Part model, mm, in its own coordinate system. A direction names the side the tool comes from. Round coordinates to 2 decimals unless told otherwise and drop trailing zeros. Write each loop counter-clockwise with the first axis right and the second up, starting at its lowest first coordinate (ties: lowest second). Pieces come first, ordered by that corner, then holes. Notation, with made-up numbers: (21.25, -6) -> (50.25, -6) arc R10 ccw to (50.25, -1) -> close; hole circle Ø5 at (18, 79). An arc over 180 degrees is marked (long way). Use CSV: the item, a comma, the result in double quotes. Start each with the question number.
(1) Saw through at A-A (z = 21.5). Give the cut face in (x, y), plus the area to 3 significant figures.
(2) Saw through at D-D (x = 0). Give the cut face in (y, z), plus the area to 3 significant figures.
(3) Two-plate mould, pull along X, no slides. Class faces 1 (the cylindrical face through (-21.664, -4.715, 12.325)), 2 (the flat face through (-25, 3, 12)), 3 (the flat face through (-0.3, -0.4, 25)): released by +X, released by -X, zero draft, split by the parting line, or undercut.
(4) Saw through at B-B (x = -20). Give the cut face in (y, z).
(5) Probe line 1 (Y direction, x = -20, z = 6.25); line 2 (X direction, y = -1.75, z = 2); line 3 (X direction, y = 3, z = 6.5). List the from-to ranges inside material, lowest first. Write a range as [from, to].
(6) Saw through at C-C (y = -1.75). Give the cut face in (x, z), plus the area to 3 significant figures.
(7) Which spindle directions (+Z, -Z, +X, -X, +Y, -Y) get a long thin tool onto all of the face, cutting with end or side? Do faces 4 (the cylindrical face through (0, -5, 15)), 5 (the cylindrical face through (0, -5, 17)), 6 (the flat face through (15, 3, 21)), 7 (the cylindrical face through (0, -7, 19)). Say none if no direction does.
(8) Drop flat-ended pins along their axis: pin 1 (2 mm diameter, centred on x = 3, y = 4.5, fed in from +Z); pin 2 (3.5 mm diameter, centred on x = -4, z = 20, fed in from +Y). Give the stop position or say it passes through.
```python
from build123d import *

# Parameters (mm, degrees)
F0_R          = 3.25
F1_DEPTH      = 25
F3_DEPTH      = 8
F4_START      = 6
F4_DEPTH      = 2
F6_DEPTH      = 25
F7_R          = 1.75
F8_DEPTH      = 25
F8_DEPTH_BACK = 25
F9_R          = 1


with BuildPart() as f1:
    # F0 (on Top) → F1 (new body)
    with BuildSketch(Plane.XY):
        with BuildLine():
            Line((-25, 6.5), (-25, 0))
            ThreePointArc((-25, 0), (-21.5811388301, -4.7434164903), (-16, -3))
            Line((-16, -3), (0, -3))
            Line((0, -3), (16, -3))
            ThreePointArc((16, -3), (21.5811388301, -4.7434164903), (25, 0))
            Line((25, 0), (25, 6.5))
            Line((25, 6.5), (-25, 6.5))
        make_face()
        with Locations((-20, 0)):
            Circle(F0_R, mode=Mode.SUBTRACT)
        with Locations((20, 0)):
            Circle(F0_R, mode=Mode.SUBTRACT)
    extrude(amount=F1_DEPTH)

    # F2 (on Front) → F3 (join)
    with BuildSketch(Plane.XZ):
        with BuildLine():
            ThreePointArc((-8, 10), (0, 15), (8, 10))
            Line((8, 10), (9.797752809, 10.8764044944))
            ThreePointArc((9.797752809, 10.8764044944), (0, 17), (-9.797752809, 10.8764044944))
            Line((-9.797752809, 10.8764044944), (-8, 10))
        make_face()
    extrude(amount=F3_DEPTH)

    # F2 (on Front) → F4 (join)
    with BuildSketch(Plane.XZ.offset(F4_START)):
        with BuildLine():
            ThreePointArc((-9.797752809, 10.8764044944), (0, 17), (9.797752809, 10.8764044944))
            Line((9.797752809, 10.8764044944), (11.595505618, 11.7528089888))
            ThreePointArc((11.595505618, 11.7528089888), (0, 19), (-11.595505618, 11.7528089888))
            Line((-11.595505618, 11.7528089888), (-9.797752809, 10.8764044944))
        make_face()
    extrude(amount=F4_DEPTH)

    # F5 (on Front) → F6 (cut)
    with BuildSketch(Plane.XZ):
        Polygon((-15, 18), (0, 18), (15, 18), (15, 26), (-15, 26), align=None)
    extrude(amount=-F6_DEPTH, mode=Mode.SUBTRACT)

    # F7 (on Front) → F8 (cut, two sides)
    with BuildSketch(Plane.XZ) as f8_sk:
        with Locations((-12, 21.5)):
            Circle(F7_R)
        with Locations((12, 21.5)):
            Circle(F7_R)
    extrude(amount=-F8_DEPTH, mode=Mode.SUBTRACT)
    extrude(f8_sk.sketch, amount=F8_DEPTH_BACK, mode=Mode.SUBTRACT)

    # F9
    f9_edges = [f1.edges().sort_by_distance(p)[0] for p in [
        (0, -3, 15),
        (-8.898876, -3, 10.438202),
        (8.898876, -3, 10.438202),
        (0, -3, 17),
        (0, -8, 15),
    ]]
    fillet(f9_edges, radius=F9_R)


solid = f1.part
```
Answers:
1,outline,"(-25, 0) arc R5 ccw to (-16, -3) -> (-13.75, -3) -> (-13.75, 0) -> (-15, 0) -> (-15, 6.5) -> (-25, 6.5) -> close; (-10.25, -3) -> (10.25, -3) -> (10.25, 0) -> (-10.25, 0) -> close; (13.75, -3) -> (16, -3) arc R5 ccw to (25, 0) -> (25, 6.5) -> (15, 6.5) -> (15, 0) -> (13.75, 0) -> close; hole circle Ø6.5 at (-20, 0); hole circle Ø6.5 at (20, 0)"
1,area,"213 mm²"
2,outline,"(-8, 16) arc R1 ccw to (-7, 15) -> (-4, 15) arc R1 cw to (-3, 14) -> (-3, 0) -> (6.5, 0) -> (6.5, 18) -> (0, 18) -> (0, 25) -> (-3, 25) -> (-3, 18) arc R1 cw to (-4, 17) -> (-6, 17) -> (-6, 19) -> (-8, 19) -> close"
2,area,"206 mm²"
3,face 1,"undercut"
3,face 2,"released by -X"
3,face 3,"zero draft"
4,outline,"(-5, 0) -> (-3.25, 0) -> (-3.25, 25) -> (-5, 25) -> close; (3.25, 0) -> (6.5, 0) -> (6.5, 25) -> (3.25, 25) -> close"
5,line 1,"y = [-5, -3.25], [3.25, 6.5]"
5,line 2,"x = [-24.68, -22.74], [-17.26, 17.26], [22.74, 24.68]"
5,line 3,"x = [-25, -21.25], [-18.75, 18.75], [21.25, 25]"
6,outline,"(-24.68, 0) -> (-22.74, 0) -> (-22.74, 25) -> (-24.68, 25) -> close; (-17.26, 0) -> (17.26, 0) -> (17.26, 25) -> (-17.26, 25) -> close; (22.74, 0) -> (24.68, 0) -> (24.68, 25) -> (22.74, 25) -> close; hole circle Ø3.5 at (-12, 21.5); hole circle Ø3.5 at (12, 21.5)"
6,area,"941 mm²"
7,face 4,"-Z, -Y"
7,face 5,"+Z"
7,face 6,"+Z, +Y"
7,face 7,"+Z, -Y"
8,pin 1,"stops at z = 18"
8,pin 2,"stops at y = 0"
